```python
from build123d import *

# Parameters (mm, degrees)
F0_R     = 3.75
F1_DEPTH = 20
F2_W     = 5.758919
F2_H     = 8.252938
F3_DEPTH = 9.4


with BuildPart() as f1:
    # F0 (on Top) → F1 (new body)
    with BuildSketch(Plane.XY):
        Circle(F0_R)
    extrude(amount=F1_DEPTH)

    # F2 (on Top) → F3 (join)
    with BuildSketch(Plane.XY):
        with Locations((2.879459, -0.073531)):
            Rectangle(F2_W, F2_H)
    extrude(amount=F3_DEPTH)

    # F4 (on Front) → F5 (revolve)
    with BuildSketch(Plane.XZ):
        Polygon((0, 30.37099), (0, 20), (3.750007, 20), align=None)
    revolve(axis=Axis((0, 0, 25.185495), (0, 0, 1)))


solid = f1.part
```
Input: part model. Units: mm. Frame: model coordinates. A direction names the side the tool comes from. Coordinates: 2 decimals unless noted, no trailing zeros. Write each loop counter-clockwise with the first axis right and the second up, starting at its lowest first coordinate (ties: lowest second). Pieces come first, ordered by that corner, then holes.
1) Pin query (flat end, axial travel): pin 1 Ø1.5 at (y, z) = (3, 24.5) entering from +X; pin 2 Ø3 at (x, z) = (1.5, 21) entering from +Y; pin 3 Ø5 at (x, z) = (3, 23) entering from -Y; pin 4 Ø4 at (y, z) = (3, 8.5) entering from -X. Return the tip coordinate at first contact, or that it passes through.
2) Section B-B on z = 26.5. Output: boundary loops of the cut face in (x, y).
3) Section A-A on z = 2. Output: boundary loops of the cut face in (x, y), and give its area (3 significant figures).
4) Set-up query: faces 1 (the flat face through (4, 0, 9.4)), 2 (the flat face through (1, 0, 0)), 3 (the cylindrical face through (-3.746, 0.165, 12.082)). Return all of +Z, -Z, +X, -X, +Y, -Y with unobstructed straight access to the full face (end or side cutting, diameter ignored); none if empty.
5) Material intervals for line 1 along Z through (x, y) = (4.25, -1); line 2 along Y through (x, z) = (-0.75, 14); line 3 along Y through (x, z) = (2, 19), sorted ascending.
Check result:
1. pin 1: passes through
1. pin 2: stops at y = 3.73
1. pin 3: stops at y = -3.07
1. pin 4: stops at x = -3.61
2. outline: circle Ø2.8 at (0, 0)
3. outline: (0, -4.2) - (5.76, -4.2) - (5.76, 4.05) - (0, 4.05) - (0, 3.75) arc R3.75 ccw to (0, -3.75) - close
3. area: 69.6 mm2
4. face 1: +Z, +X
4. face 2: -Z, +X, -X, +Y, -Y
4. face 3: +Z
5. line 1: z = 0 to 9.4
5. line 2: y = -3.67 to 3.67
5. line 3: y = -3.17 to 3.17
